Here's how the part is built. I have some questions about the finished solid (model axes, mm). Round coordinates to 2 decimals unless told otherwise and drop trailing zeros. Loops run counter-clockwise (first coordinate to the right, second up) from the corner with the lowest first, then second, coordinate; pieces in that order, holes last. Notation, with made-up numbers: M -9,54.25 L 33,54.25 A25 ccw 33,85.25 Z; hole C -28,-17 d9. An arc over 180 degrees is marked long. Write item = value, one per line. Start each with the question number.
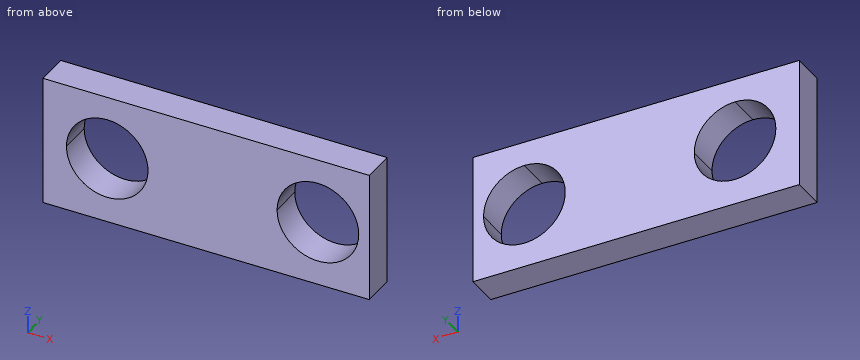
from build123d import *

# Parameters (mm, degrees)
SKETCH1_W           = 127
SKETCH1_H           = 50.8
BOSS_EXTRUDE1_DEPTH = 12.7
CUT_EXTRUDE1_DEPTH  = 12.7
CUT_EXTRUDE2_DEPTH  = 13.7


with BuildPart() as part:
    # Sketch1 → Boss-Extrude1 (new body)
    with BuildSketch(Plane(origin=(0, 0, 0), x_dir=(1, 0, 0), z_dir=(0, 1, 0))):
        with Locations((63.5, 25.4)):
            Rectangle(SKETCH1_W, SKETCH1_H)
    extrude(amount=BOSS_EXTRUDE1_DEPTH)

    # Sketch2 → Cut-Extrude1 (cut)
    with BuildSketch(Plane(origin=(0, 12.7, 0), x_dir=(1, 0, 0), z_dir=(0, 1, 0))):
        with BuildLine():
            ThreePointArc((9.125, 25), (13.774679849, 13.774679849), (25, 9.125))
            Line((25, 9.125), (25, 25))
            Line((25, 25), (9.125, 25))
        make_face()
        with BuildLine():
            Line((25, 25), (25, 9.125))
            ThreePointArc((25, 9.125), (36.225320151, 13.774679849), (40.875, 25))
            ThreePointArc((40.875, 25), (25, 40.875), (9.125, 25))
            Line((9.125, 25), (25, 25))
        make_face()
    extrude(amount=-CUT_EXTRUDE1_DEPTH, mode=Mode.SUBTRACT)

    # Sketch4 → Cut-Extrude2 (cut, through all)
    with BuildSketch(Plane(origin=(0, 12.7, 0), x_dir=(1, 0, 0), z_dir=(0, 1, 0))):
        with BuildLine():
            ThreePointArc((91.1, 25.4), (95.757002179, 14.157002179), (107, 9.5))
            Line((107, 9.5), (107, 25.4))
            Line((107, 25.4), (91.1, 25.4))
        make_face()
        with BuildLine():
            Line((107, 25.4), (107, 9.5))
            ThreePointArc((107, 9.5), (118.242997821, 14.157002179), (122.9, 25.4))
            ThreePointArc((122.9, 25.4), (107, 41.3), (91.1, 25.4))
            Line((91.1, 25.4), (107, 25.4))
        make_face()
    extrude(amount=-CUT_EXTRUDE2_DEPTH, mode=Mode.SUBTRACT)


solid = part.part
Item 1: I want a section at C-C, the plane x = 114.5. List the corners of the cut face in (y, z) for me.
Item 2: I want a section at A-A, the plane y = 6.25. List the corners of the cut face in (x, z) for me (3 decimals), then the cut area to 3 significant figures.
Item 3: I want a section at D-D, the plane x = 19.5. List the corners of the cut face in (y, z) for me, then the cut area to 3 significant figures.
Item 4: Will this pin go through, and if not, where does the flat tip stop? pin 1 Ø2 at (x, z) = (98, -36) entering from +Y.
Item 5: I want a section at B-B, the plane z = -15. List the corners of the cut face in (x, y) for me, then the cut area to 3 significant figures.
Item 6: Please list where these lines run through material, in increasing order: line 1 (X direction, y = 11.25, z = -25.5); line 2 (X direction, y = 4.25, z = -34.5); line 3 (Z direction, x = 106.5, y = 1). Write a range as [from, to].
Worked out:
q1.outline = M 0,-50.8 L 12.7,-50.8 L 12.7,-39.42 L 0,-39.42 Z; M 0,-11.38 L 12.7,-11.38 L 12.7,0 L 0,0 Z
q2.outline = M 0,-50.8 L 127,-50.8 L 127,0 L 0,0 Z; hole C 25,-25 d31.75; hole C 107,-25.4 d31.8
q2.area = 4,870 mm2
q3.outline = M 0,-50.8 L 12.7,-50.8 L 12.7,-39.89 L 0,-39.89 Z; M 0,-10.11 L 12.7,-10.11 L 12.7,0 L 0,0 Z
q3.area = 267 mm2
q4.pin_1 = through
q5.outline = M 0,0 L 12.67,0 L 12.67,12.7 L 0,12.7 Z; M 37.33,0 L 94.97,0 L 94.97,12.7 L 37.33,12.7 Z; M 119.03,0 L 127,0 L 127,12.7 L 119.03,12.7 Z
q5.area = 994 mm2
q6.line_1 = [0, 9.13], [40.87, 91.1], [122.9, 127]
q6.line_2 = [0, 12.28], [37.72, 93.96], [120.04, 127]
q6.line_3 = [-50.8, -41.29], [-9.51, 0]
